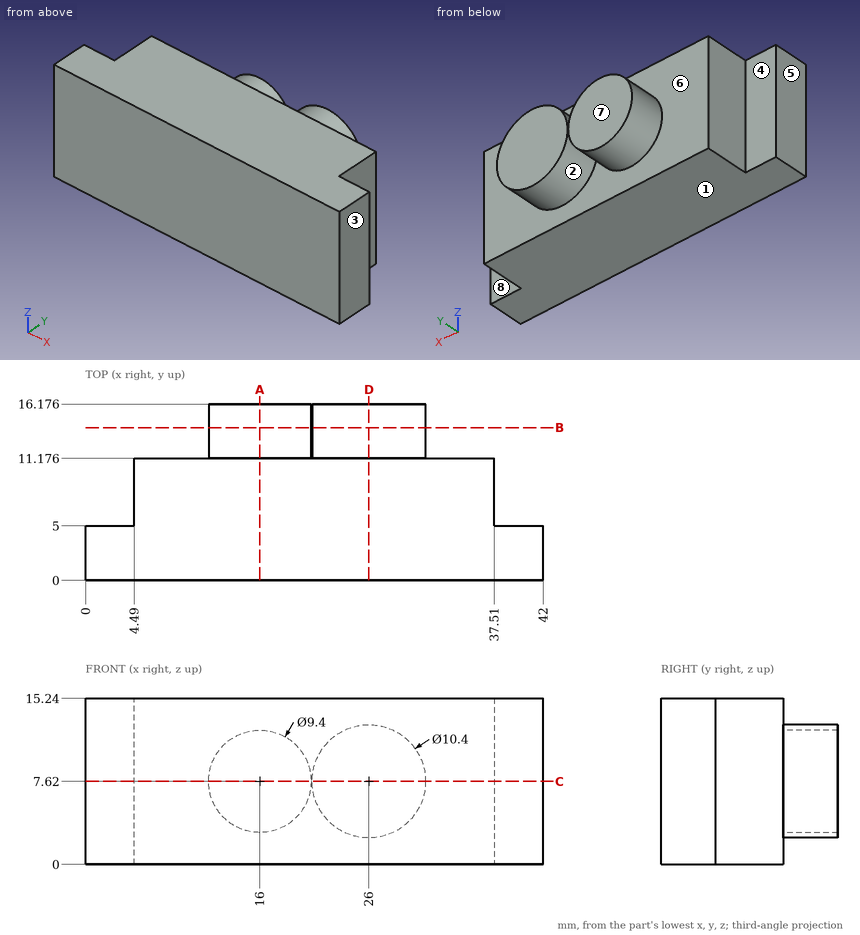
The figure shows three views and two pictorial views of one solid part (mm, origin at its lowest corner). Answer the questions. A direction names the side the tool comes from. Give positions to 0.01 mm unless a question says otherwise; leave off trailing zeros. Write each loop counter-clockwise with the first axis right and the second up, starting at its lowest first coordinate (ties: lowest second). Pieces come first, ordered by that corner, then holes. Notation, with made-up numbers: (59, 49.5) -> (95, 49.5) arc R15 ccw to (95, 54.5) -> close; hole circle Ø8 at (80, -7). An arc over 180 degrees is marked (long way). Write each question's results on one line, items separated by ' | '.
1. Find section D-D on x = 26. Determine the outline of the cut face in (y, z).
Data:
outline: (0, 0) -> (11.18, 0) -> (11.18, 2.42) -> (16.18, 2.42) -> (16.18, 12.82) -> (11.18, 12.82) -> (11.18, 15.24) -> (0, 15.24) -> close
2. Each of these flat-tipped pins is pushed along its axis until it touches: pin 1 Ø1.5 at (y, z) = (8.5, 2) entering from +X; pin 2 Ø3 at (y, z) = (13, 12.5) entering from +X; pin 3 Ø6 at (y, z) = (14.5, 2.5) entering from -X. Where does it stop, or does it pass through?
Data:
pin 1: x = 37.51 | pin 2: x = 29.95 | pin 3: x = 11.81
3. Straight lines are drawn through the part: L1, parallel to Y at x = 40.5, z = 9.5; L2, parallel to Y at x = 11.5, z = 3.75; L3, parallel to X at y = 6, z = 5. For each, find the intervals that lie inside material, in ascending order.
Data:
L1: 0 to 5 | L2: 0 to 11.18 | L3: 4.49 to 37.51
4. Determine the mould class of the marked faces 1, 2 and 3 for opening direction X: +X half, -X half, draft (parallel to the pull), parting line (faces both ways), or undercut.
Data:
face 1: draft | face 2: undercut | face 3: +X half
5. A tool of negligible diameter and unlimited length cuts with its end or side. For the marked faces 4, 5, 6, 7 and 8, from which of +Z, -Z, +X, -X, +Y, -Y can it reach the whole face along a straight path? Write none if from no direction.
Data:
face 4: +Z, -Z, -X, +Y | face 5: +Z, -Z, -X, +Y, -Y | face 6: +Y | face 7: +Z, -Z, +X, -X, +Y | face 8: +Z, -Z, +X, +Y
6. Find section B-B on y = 14. Determine the outline of the cut face in (x, z).
Data:
outline: circle Ø9.4 at (16, 7.62); circle Ø10.4 at (26, 7.62)
7. Find section C-C on z = 7.62. Determine the outline of the cut face in (x, y).
Data:
outline: (0, 0) -> (42, 0) -> (42, 5) -> (37.51, 5) -> (37.51, 11.18) -> (31.2, 11.18) -> (31.2, 16.18) -> (20.8, 16.18) -> (20.8, 11.18) -> (20.7, 11.18) -> (20.7, 16.18) -> (11.3, 16.18) -> (11.3, 11.18) -> (4.49, 11.18) -> (4.49, 5) -> (0, 5) -> close
8. Find section A-A on x = 16. Determine the outline of the cut face in (y, z).
Data:
outline: (0, 0) -> (11.18, 0) -> (11.18, 2.92) -> (16.18, 2.92) -> (16.18, 12.32) -> (11.18, 12.32) -> (11.18, 15.24) -> (0, 15.24) -> close
